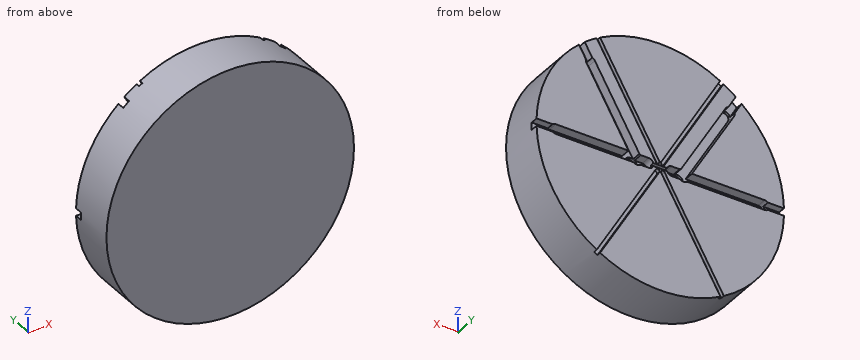
from build123d import *

# Parameters (mm, degrees)
SKETCH1_R           = 8
BOSS_EXTRUDE1_DEPTH = 3
CUT_EXTRUDE1_DEPTH  = 0.25
SKETCH3_R           = 0.4
CUT_EXTRUDE2_DEPTH  = 0.8
CUT_EXTRUDE4_DEPTH  = 0.635
CUT_EXTRUDE6_DEPTH  = 0.48


with BuildPart() as part:
    # Sketch1 → Boss-Extrude1 (new body)
    with BuildSketch(Plane(origin=(0, 0, 0), x_dir=(1, 0, 0), z_dir=(0, 1, 0))):
        Circle(SKETCH1_R)
    extrude(amount=-BOSS_EXTRUDE1_DEPTH)

    # Sketch2 → Cut-Extrude1 (cut)
    with BuildSketch(Plane(origin=(0, 0, 0), x_dir=(1, 0, 0), z_dir=(0, 1, 0))):
        with BuildLine():
            Line((-0.75, 0.1), (0.75, 0.1))
            ThreePointArc((0.75, 0.1), (0.85, 0), (0.75, -0.1))
            Line((0.75, -0.1), (-0.75, -0.1))
            ThreePointArc((-0.75, -0.1), (-0.85, 0), (-0.75, 0.1))
        make_face()
        with BuildLine():
            Line((0.064947675, 0.362501474), (4.891747675, 8.722501474))
            ThreePointArc((4.891747675, 8.722501474), (5.062501474, 8.768252325), (5.108252325, 8.597498526))
            Line((5.108252325, 8.597498526), (0.281452325, 0.237498526))
            ThreePointArc((0.281452325, 0.237498526), (0.110698526, 0.191747675), (0.064947675, 0.362501474))
        make_face()
        with BuildLine():
            Line((0.281452325, -0.237498526), (5.108252325, -8.597498526))
            ThreePointArc((5.108252325, -8.597498526), (5.062501474, -8.768252325), (4.891747675, -8.722501474))
            Line((4.891747675, -8.722501474), (0.064947675, -0.362501474))
            ThreePointArc((0.064947675, -0.362501474), (0.110698526, -0.191747675), (0.281452325, -0.237498526))
        make_face()
        with BuildLine():
            Line((-0.064747026, -0.362152654), (-4.891547026, -8.784654127))
            ThreePointArc((-4.891547026, -8.784654127), (-5.062152654, -8.830954448), (-5.108452974, -8.66034882))
            Line((-5.108452974, -8.66034882), (-0.281652974, -0.237847346))
            ThreePointArc((-0.281652974, -0.237847346), (-0.111047346, -0.191547026), (-0.064747026, -0.362152654))
        make_face()
        with BuildLine():
            Line((-0.281452325, 0.237498526), (-5.108252325, 8.597498526))
            ThreePointArc((-5.108252325, 8.597498526), (-5.062501474, 8.768252325), (-4.891747675, 8.722501474))
            Line((-4.891747675, 8.722501474), (-0.064947675, 0.362501474))
            ThreePointArc((-0.064947675, 0.362501474), (-0.110698526, 0.191747675), (-0.281452325, 0.237498526))
        make_face()
    extrude(amount=-CUT_EXTRUDE1_DEPTH, mode=Mode.SUBTRACT)

    # Sketch3 → Cut-Extrude2 (cut)
    with BuildSketch(Plane(origin=(0, 0, 0), x_dir=(1, 0, 0), z_dir=(0, 1, 0))):
        with Locations((1.5, 0)):
            Circle(SKETCH3_R)
        with Locations((-1.5, 0)):
            Circle(SKETCH3_R)
    extrude(amount=-CUT_EXTRUDE2_DEPTH, mode=Mode.SUBTRACT)

    # Sketch4 → Cut-Extrude4 (cut)
    with BuildSketch(Plane(origin=(0, 0, 0), x_dir=(1, 0, 0), z_dir=(0, 1, 0))):
        with BuildLine():
            Line((-0.75, -0.3175), (-6.75, -0.3175))
            ThreePointArc((-6.75, -0.3175), (-7.0675, 0), (-6.75, 0.3175))
            Line((-6.75, 0.3175), (-0.75, 0.3175))
            ThreePointArc((-0.75, 0.3175), (-0.4325, 0), (-0.75, -0.3175))
        make_face()
        with BuildLine():
            Line((0.75, 0.3175), (6.75, 0.3175))
            ThreePointArc((6.75, 0.3175), (7.0675, 0), (6.75, -0.3175))
            Line((6.75, -0.3175), (0.75, -0.3175))
            ThreePointArc((0.75, -0.3175), (0.4325, 0), (0.75, 0.3175))
        make_face()
        with BuildLine():
            Line((-1.225038951, -0.158753493), (-4.225104953, -5.354867808))
            ThreePointArc((-4.225104953, -5.354867808), (-4.658819495, -5.471075365), (-4.775027051, -5.037360823))
            Line((-4.775027051, -5.037360823), (-1.774961049, 0.158753493))
            ThreePointArc((-1.774961049, 0.158753493), (-1.341246507, 0.274961049), (-1.225038951, -0.158753493))
        make_face()
        with BuildLine():
            Line((1.774961049, 0.158753493), (4.775027051, -5.037360823))
            ThreePointArc((4.775027051, -5.037360823), (4.658819495, -5.471075365), (4.225104953, -5.354867808))
            Line((4.225104953, -5.354867808), (1.225038951, -0.158753493))
            ThreePointArc((1.225038951, -0.158753493), (1.341246507, 0.274961049), (1.774961049, 0.158753493))
        make_face()
    extrude(amount=-CUT_EXTRUDE4_DEPTH, mode=Mode.SUBTRACT)

    # Sketch5 → Cut-Extrude6 (cut)
    with BuildSketch(Plane(origin=(0, 0, 0), x_dir=(1, 0, 0), z_dir=(0, 1, 0))):
        with BuildLine():
            Line((-6.75, -0.24), (-8.75, -0.24))
            ThreePointArc((-8.75, -0.24), (-8.99, 0), (-8.75, 0.24))
            Line((-8.75, 0.24), (-6.75, 0.24))
            ThreePointArc((-6.75, 0.24), (-6.51, 0), (-6.75, -0.24))
        make_face()
        with BuildLine():
            Line((6.75, 0.24), (8.75, 0.24))
            ThreePointArc((8.75, 0.24), (8.99, 0), (8.75, -0.24))
            Line((8.75, -0.24), (6.75, -0.24))
            ThreePointArc((6.75, -0.24), (6.51, 0), (6.75, 0.24))
        make_face()
        with BuildLine():
            Line((-4.29222143, -5.316116956), (-6.844144056, -9.736046945))
            ThreePointArc((-6.844144056, -9.736046945), (-7.171991269, -9.823888878), (-7.259833201, -9.496041665))
            Line((-7.259833201, -9.496041665), (-4.707910575, -5.076111676))
            ThreePointArc((-4.707910575, -5.076111676), (-4.380063362, -4.988269743), (-4.29222143, -5.316116956))
        make_face()
        with BuildLine():
            Line((4.707910575, -5.076111676), (7.190547612, -9.376039025))
            ThreePointArc((7.190547612, -9.376039025), (7.10270568, -9.703886238), (6.774858467, -9.616044305))
            Line((6.774858467, -9.616044305), (4.29222143, -5.316116956))
            ThreePointArc((4.29222143, -5.316116956), (4.380063362, -4.988269743), (4.707910575, -5.076111676))
        make_face()
    extrude(amount=-CUT_EXTRUDE6_DEPTH, mode=Mode.SUBTRACT)


solid = part.part
Can you work these out from the model? Positions are in its coordinate system, mm. Give positions to 0.01 mm unless a question says otherwise; leave off trailing zeros. Order: outer loops, then holes, each group sorted by start corner. A loop starts at its lowest first (then second) coordinate and runs counter-clockwise, first axis right, second up. Notation, with made-up numbers: M -18,-24 L 24,-24 A3 ccw 24,-19 Z; hole C -28,79.5 d4. An arc over 180 degrees is marked long. One line per item, written item: value.
Item 1: If we section it at C-C on z = 2.25: Write out the boundary of the cut face in (x, y) (3 decimals).
Verdict:
outline: M -7.677,-3 L 7.677,-3 L 7.677,0 L 3.166,0 L 3.166,-0.635 L 2.432,-0.635 L 2.432,0 L 1.443,0 L 1.443,-0.25 L 1.155,-0.25 L 1.155,0 L -1.147,0 L -1.147,-0.25 L -1.435,-0.25 L -1.435,0 L -2.432,0 L -2.432,-0.635 L -3.166,-0.635 L -3.166,0 L -7.677,0 Z
Item 2: If we section it at A-A on z = -3.5: Write out the boundary of the cut face in (x, y), and give its area (3 significant figures).
Verdict:
outline: M -7.19,-3 L 7.19,-3 L 7.19,0 L 2.17,0 L 2.17,-0.25 L 1.88,-0.25 L 1.88,0 L -1.88,0 L -1.88,-0.25 L -2.17,-0.25 L -2.17,0 L -7.19,0 Z
area: 43.0 mm2
Item 3: Please list where these lines run through material, in increasing order: line 1 (X direction, y = -0.55, z = 0); line 2 (Z direction, x = -0.25, y = -2.55).
Verdict:
line 1: -8 to -7.07, -0.43 to 0.43, 7.07 to 8
line 2: -8 to 8
Item 4: For pin 1 (3 mm diameter, centred on x = -5.5, z = -6, fed in from -Y); pin 2 (0.5 mm diameter, centred on x = -7.5, y = -0.5, fed in from -Z); pin 3 (0.6 mm diameter, centred on x = 1.5, z = 0, fed in from +Y); pin 4 (1.5 mm diameter, centred on x = 2.5, y = -1, fed in from -Z), each with a flat end and sliding along its axis, tell me the tip position at first contact or that it passes through.
Verdict:
pin 1: y = -3
pin 2: z = -3.38
pin 3: y = -0.8
pin 4: z = -7.81
Item 5: If we section it at B-B on y = -1.75: Write out the boundary of the cut face in (x, z).
Verdict:
outline: C 0,0 d16
